```python
from build123d import *

# Parameters (mm, degrees)
SKIZZE1_W                       = 62.5
SKIZZE1_H                       = 82.5
AUFSATZ_LINEAR_AUSTRAGEN1_DEPTH = 4
AUFSATZ_LINEAR_START            = -4
SKIZZE2_W                       = 5
SKIZZE2_H                       = 5
SKIZZE2_R                       = 1.25
AUFSATZ_LINEAR_AUSTRAGEN2_DEPTH = 4
SKIZZE3_W                       = 62.5
SKIZZE3_H                       = 82.5
AUFSATZ_LINEAR_AUSTRAGEN3_DEPTH = 2
SKIZZE2_2_R                     = 1.25
SCHNITT_LINEAR_AUSTRAGEN1_DEPTH = 5
SCHNITT_LINEAR_START            = -2
SKIZZE4_R                       = 1.25
SCHNITT_LINEAR_AUSTRAGEN2_DEPTH = 2
SKIZZE5_W                       = 12.5
SKIZZE5_H                       = 2
SCHNITT_LINEAR_AUSTRAGEN3_DEPTH = 4


with BuildPart() as part:
    # Skizze1 → Aufsatz-Linear austragen1 (new body)
    with BuildSketch(Plane.XY):
        with Locations((1.25, -6.25)):
            Rectangle(SKIZZE1_W, SKIZZE1_H)
        with BuildLine():
            ThreePointArc((-28, 31.354356), (-26.616117, 31.616117), (-26.354356, 33))
            Line((-26.354356, 33), (28.854356, 33))
            ThreePointArc((28.854356, 33), (29.116117, 31.616117), (30.5, 31.354356))
            Line((30.5, 31.354356), (30.5, -43.854356))
            ThreePointArc((30.5, -43.854356), (29.116117, -44.116117), (28.854356, -45.5))
            Line((28.854356, -45.5), (-26.354356, -45.5))
            ThreePointArc((-26.354356, -45.5), (-26.616117, -44.116117), (-28, -43.854356))
            Line((-28, -43.854356), (-28, 31.354356))
        make_face(mode=Mode.SUBTRACT)
    extrude(amount=AUFSATZ_LINEAR_AUSTRAGEN1_DEPTH)

    # Skizze2 → Aufsatz-Linear austragen2 (add)
    # profile 1 of 4: a face of its own
    with BuildSketch(Plane.XY.offset(4).offset(AUFSATZ_LINEAR_START)):
        with Locations((-27.5, -45)):
            Rectangle(SKIZZE2_W, SKIZZE2_H)
        with Locations((-27.5, -45)):
            Circle(SKIZZE2_R, mode=Mode.SUBTRACT)
    # profile 2 of 4: a face of its own
    with BuildSketch(Plane.XY.offset(4).offset(AUFSATZ_LINEAR_START)):
        with Locations((30, -45)):
            Rectangle(SKIZZE2_W, SKIZZE2_H)
        with Locations((30, -45)):
            Circle(SKIZZE2_R, mode=Mode.SUBTRACT)
    # profile 3 of 4: a face of its own
    with BuildSketch(Plane.XY.offset(4).offset(AUFSATZ_LINEAR_START)):
        with Locations((30, 32.5)):
            Rectangle(SKIZZE2_W, SKIZZE2_H)
        with Locations((30, 32.5)):
            Circle(SKIZZE2_R, mode=Mode.SUBTRACT)
    # profile 4 of 4: a face of its own
    with BuildSketch(Plane.XY.offset(4).offset(AUFSATZ_LINEAR_START)):
        with Locations((-27.5, 32.5)):
            Rectangle(SKIZZE2_W, SKIZZE2_H)
        with Locations((-27.5, 32.5)):
            Circle(SKIZZE2_R, mode=Mode.SUBTRACT)
    extrude(amount=AUFSATZ_LINEAR_AUSTRAGEN2_DEPTH)

    # Skizze3 → Aufsatz-Linear austragen3 (add)
    with BuildSketch(Plane.XY.offset(4)):
        with Locations((1.25, -6.25)):
            Rectangle(SKIZZE3_W, SKIZZE3_H)
    extrude(amount=AUFSATZ_LINEAR_AUSTRAGEN3_DEPTH)

    # Skizze2<2> → Schnitt-Linear austragen1 (cut)
    with BuildSketch(Plane.XY.offset(4)):
        with BuildLine():
            ThreePointArc((-26.354356, -45.5), (-26.276367, -45.255387), (-26.25, -45))
            ThreePointArc((-26.25, -45), (-26.815347, -43.954175), (-28, -43.854356))
            ThreePointArc((-28, -43.854356), (-28.383883, -45.883883), (-26.354356, -45.5))
        make_face()
        with BuildLine():
            ThreePointArc((30.5, 31.354356), (31.045825, 31.815347), (31.25, 32.5))
            ThreePointArc((31.25, 32.5), (30.255387, 33.723633), (28.854356, 33))
            ThreePointArc((28.854356, 33), (29.116117, 31.616117), (30.5, 31.354356))
        make_face()
        with BuildLine():
            ThreePointArc((-28, 31.354356), (-26.815347, 31.454175), (-26.25, 32.5))
            ThreePointArc((-26.25, 32.5), (-26.276367, 32.755387), (-26.354356, 33))
            ThreePointArc((-26.354356, 33), (-28.383883, 33.383883), (-28, 31.354356))
        make_face()
        with Locations((30, -45)):
            Circle(SKIZZE2_2_R)
    extrude(amount=-SCHNITT_LINEAR_AUSTRAGEN1_DEPTH, mode=Mode.SUBTRACT)

    # Skizze4 → Schnitt-Linear austragen2 (cut)
    with BuildSketch(Plane(origin=(0, 0, 4), x_dir=(-1, 0, 0), z_dir=(0, 0, -1)).offset(SCHNITT_LINEAR_START)):
        with Locations(Location((27.5, 32.5, 0), (0, 0, 180))):
            Circle(SKIZZE4_R)
        with Locations(Location((27.5, -45, 0), (0, 0, 180))):
            Circle(SKIZZE4_R)
        with Locations(Location((-30, -45, 0), (0, 0, 180))):
            Circle(SKIZZE4_R)
        with Locations(Location((-30, 32.5, 0), (0, 0, 180))):
            Circle(SKIZZE4_R)
    extrude(amount=SCHNITT_LINEAR_AUSTRAGEN2_DEPTH, mode=Mode.SUBTRACT)

    # Skizze5 → Schnitt-Linear austragen3 (cut)
    with BuildSketch(Plane(origin=(0, 0, 0), x_dir=(-1, 0, 0), z_dir=(0, 0, -1))):
        with Locations((-1.25, -46.5)):
            Rectangle(SKIZZE5_W, SKIZZE5_H)
    extrude(amount=-SCHNITT_LINEAR_AUSTRAGEN3_DEPTH, mode=Mode.SUBTRACT)


solid = part.part
```
Model file for the job. Use its own axes, mm. A direction names the side the tool comes from. Coordinates: 2 decimals unless noted, no trailing zeros. Order: outer loops, then holes, each group sorted by start corner. A loop starts at its lowest first (then second) coordinate and runs counter-clockwise, first axis right, second up. Notation, with made-up numbers: (66.25, 39) -> (122.25, 39) arc R9 ccw to (122.25, 56) -> close; hole circle Ø3 at (57.5, 31.5). An arc over 180 degrees is marked (long way). Answer as a JSON object with one key per item and string values. Group by question number.
1) Pull direction Y, two halves, no side cores. Call faces 4 (the face through (18, -45.5, 2)), 5 (the face through (0.8, -47.5, 4.3)), 6 (the face through (-29, -3, 0)): +Y half, -Y half, draft (parallel to the pull), parting line (faces both ways), or undercut.
2) Flat gauge pins, fed straight in: pin 1 (12 mm diameter, centred on x = -19.5, y = -32.5, fed in from -Z); pin 2 (2 mm diameter, centred on x = -27.5, y = 32.5, fed in from +Z). Where does each tip first touch, or does it go through?
3) Which spindle directions (+Z, -Z, +X, -X, +Y, -Y) get a long thin tool onto all of the face, cutting with end or side? Do faces 1 (the face through (-27, 30, 2)), 2 (the face through (-5, -47, 2)), 3 (the face through (1, 35, 3)). Say none if no direction does.
4) Drill centre lines: L1, parallel to X at y = 32.5, z = 2.5; L2, parallel to Y at x = -27.5, z = 1.25; L3, parallel to Y at x = -27.5, z = 5.35. Where is each one in solid material? Low to high.
5) Cut at B-B, the plane y = 14. Write the cut outline in (x, z), then the cut area to 3 significant figures.
6) Cut at A-A, the plane z = 2.15. Write the cut outline in (x, y).
7) Cut at C-C, the plane x = -21. Write the cut outline in (y, z), then the cut area to 3 significant figures.
Check values:
{
 "1": {"face 4": "undercut", "face 5": "-Y half", "face 6": "draft"},
 "2": {"pin 1": "stops at z = 4", "pin 2": "passes through"},
 "3": {"face 1": "-Z", "face 2": "-Z, -Y", "face 3": "+Z, -Z, +X, -X, +Y"},
 "4": {"L1": "x = -30 to -28.75, -26.25 to -25, 27.5 to 28.75, 31.25 to 32.5", "L2": "y = -47.5 to -46.25, -43.75 to -42.5, 30 to 31.25, 33.75 to 35", "L3": "y = -47.5 to -46.25, -43.75 to 31.25, 33.75 to 35"},
 "5": {"outline": "(-30, 0) -> (-28, 0) -> (-28, 4) -> (30.5, 4) -> (30.5, 0) -> (32.5, 0) -> (32.5, 6) -> (-30, 6) -> close", "area": "141 mm²"},
 "6": {"outline": "(-30, -47.5) -> (-5, -47.5) -> (-5, -45.5) -> (-25, -45.5) -> (-25, -42.5) -> (-28, -42.5) -> (-28, 30) -> (-25, 30) -> (-25, 33) -> (27.5, 33) -> (27.5, 30) -> (30.5, 30) -> (30.5, -42.5) -> (27.5, -42.5) -> (27.5, -45.5) -> (7.5, -45.5) -> (7.5, -47.5) -> (32.5, -47.5) -> (32.5, 35) -> (-30, 35) -> close; hole circle Ø2.5 at (-27.5, -45); hole circle Ø2.5 at (-27.5, 32.5); hole circle Ø2.5 at (30, -45); hole circle Ø2.5 at (30, 32.5)"},
 "7": {"outline": "(-47.5, 0) -> (-45.5, 0) -> (-45.5, 4) -> (33, 4) -> (33, 0) -> (35, 0) -> (35, 6) -> (-47.5, 6) -> close", "area": "181 mm²"}
}
